Build history of the part. All positions in model axes, mm. A direction names the side the tool comes from. Give positions to 0.01 mm unless a question says otherwise; leave off trailing zeros. Order: outer loops, then holes, each group sorted by start corner. A loop starts at its lowest first (then second) coordinate and runs counter-clockwise, first axis right, second up. Notation, with made-up numbers: (-10, 34.5) - (24, 34.5) arc R17 ccw to (24, 63.5) - close; hole circle Ø1 at (15, 82). An arc over 180 degrees is marked (long way). Use a Markdown table: item, result.
from build123d import *

# Parameters (mm, degrees)
SKETCH_W          = 53.23309
SKETCH_H          = 53.233089
PAD_DEPTH         = 19
SKETCH001_R       = 3.8
POCKET_DEPTH      = 2.001
POCKET_DEPTH_BACK = -17.001
SKETCH002_W       = 57.23309
SKETCH002_H       = 57.233089
SKETCH002_W_2     = 53.23309
SKETCH002_H_2     = 53.233089
PAD001_DEPTH      = 22


with BuildPart() as part:
    # Sketch → Pad (new body)
    with BuildSketch(Plane.XY):
        with Locations((-20.099382, 19.900122)):
            Rectangle(SKETCH_W, SKETCH_H)
    extrude(amount=PAD_DEPTH)

    # Sketch001 (on Sketch) → Pocket (cut, two sides)
    with BuildSketch(Plane.XY.offset(2)) as pocket_sk:
        Circle(SKETCH001_R)
        with Locations((-9.999876, -0.049815)):
            Circle(SKETCH001_R)
        with Locations((-19.999752, -0.09963)):
            Circle(SKETCH001_R)
        with Locations((-29.999628, -0.149445)):
            Circle(SKETCH001_R)
        with Locations((-39.999504, -0.19926)):
            Circle(SKETCH001_R)
        with Locations((-0.049815, 9.999876)):
            Circle(SKETCH001_R)
        with Locations((-10.049691, 9.950061)):
            Circle(SKETCH001_R)
        with Locations((-20.049567, 9.900246)):
            Circle(SKETCH001_R)
        with Locations((-30.049443, 9.850431)):
            Circle(SKETCH001_R)
        with Locations((-40.049319, 9.800616)):
            Circle(SKETCH001_R)
        with Locations((-0.09963, 19.999752)):
            Circle(SKETCH001_R)
        with Locations((-10.099506, 19.949937)):
            Circle(SKETCH001_R)
        with Locations((-20.099382, 19.900122)):
            Circle(SKETCH001_R)
        with Locations((-30.099258, 19.850307)):
            Circle(SKETCH001_R)
        with Locations((-40.099134, 19.800492)):
            Circle(SKETCH001_R)
        with Locations((-0.149445, 29.999628)):
            Circle(SKETCH001_R)
        with Locations((-10.149321, 29.949813)):
            Circle(SKETCH001_R)
        with Locations((-20.149197, 29.899998)):
            Circle(SKETCH001_R)
        with Locations((-30.149073, 29.850183)):
            Circle(SKETCH001_R)
        with Locations((-40.148949, 29.800368)):
            Circle(SKETCH001_R)
        with Locations((-0.19926, 39.999504)):
            Circle(SKETCH001_R)
        with Locations((-10.199136, 39.949689)):
            Circle(SKETCH001_R)
        with Locations((-20.199012, 39.899874)):
            Circle(SKETCH001_R)
        with Locations((-30.198888, 39.850059)):
            Circle(SKETCH001_R)
        with Locations((-40.198764, 39.800244)):
            Circle(SKETCH001_R)
    extrude(amount=-POCKET_DEPTH, mode=Mode.SUBTRACT)
    extrude(pocket_sk.sketch, amount=-POCKET_DEPTH_BACK, mode=Mode.SUBTRACT)

    # Sketch002 → Pad001 (join)
    with BuildSketch(Plane.XY):
        with Locations((-20.099382, 19.900122)):
            Rectangle(SKETCH002_W, SKETCH002_H)
        with Locations((-20.099382, 19.900122)):
            Rectangle(SKETCH002_W_2, SKETCH002_H_2, mode=Mode.SUBTRACT)
    extrude(amount=PAD001_DEPTH)


solid = part.part
1) Slice it at A-A (x = -42.5). Write the cut outline in (y, z).
Computed:
| item | result |
|---|---|
| outline | (-8.72, 0) - (-3.06, 0) - (-3.06, 19) - (-6.72, 19) - (-6.72, 22) - (-8.72, 22) - close; (2.66, 0) - (6.9, 0) - (6.9, 19) - (2.66, 19) - close; (12.7, 0) - (16.86, 0) - (16.86, 19) - (12.7, 19) - close; (22.75, 0) - (26.81, 0) - (26.81, 19) - (22.75, 19) - close; (32.79, 0) - (36.78, 0) - (36.78, 19) - (32.79, 19) - close; (42.82, 0) - (48.52, 0) - (48.52, 22) - (46.52, 22) - (46.52, 19) - (42.82, 19) - close |
2) Two-plate mould, pull along Y, no slides. Class faces 3 (the cylindrical face through (-40.54, 13.57, 9.63)), 4 (the flat face through (-21, 48.517, 11)), 5 (the flat face through (-22, -8, 22)): +Y half, -Y half, draft (parallel to the pull), parting line (faces both ways), or undercut.
Computed:
| item | result |
|---|---|
| face 3 | undercut |
| face 4 | +Y half |
| face 5 | draft |
3) Wall check: line 1 (Y direction, x = -20, z = 5); line 2 (Y direction, x = -40, z = 12); line 3 (X direction, y = 31.5, z = 21). Give the ranges that are in metal, low to high. Write a range as from..to.
Computed:
| item | result |
|---|---|
| line 1 | y = -8.72..-3.9, 3.7..6.1, 13.7..16.1, 23.7..26.1, 33.7..36.11, 43.69..48.52 |
| line 2 | y = -8.72..-4, 3.6..6, 13.6..16, 23.6..26, 33.6..36.01, 43.6..48.52 |
| line 3 | x = -48.72..-46.72, 6.52..8.52 |
4) Pin check, flat tips, straight feed: P1, Ø12, axis at x = -10.2, y = 39.95, coming from the +Z side; P2, Ø6, axis at x = -10.05, y = 9.95, coming from the -Z side. Stop position of each tip, or through.
Computed:
| item | result |
|---|---|
| P1 | stops at z = 19 |
| P2 | passes through |
5) Tool access for faces 1 (the cylindrical face through (-3.796, 0.167, 9.633)), 2 (the flat face through (-46.716, 20, 20)): list every direction of +Z, -Z, +X, -X, +Y, -Y with a clear straight run to the whole face (end or side of a thin tool).
Computed:
| item | result |
|---|---|
| face 1 | +Z, -Z |
| face 2 | +Z |
6) Slice it at C-C (y = -1). Write the cut outline in (x, z).
Computed:
| item | result |
|---|---|
| outline | (-48.72, 0) - (-43.71, 0) - (-43.71, 19) - (-46.72, 19) - (-46.72, 22) - (-48.72, 22) - close; (-36.28, 0) - (-33.7, 0) - (-33.7, 19) - (-36.28, 19) - close; (-26.3, 0) - (-23.69, 0) - (-23.69, 19) - (-26.3, 19) - close; (-16.31, 0) - (-13.68, 0) - (-13.68, 19) - (-16.31, 19) - close; (-6.32, 0) - (-3.67, 0) - (-3.67, 19) - (-6.32, 19) - close; (3.67, 0) - (8.52, 0) - (8.52, 22) - (6.52, 22) - (6.52, 19) - (3.67, 19) - close |
7) Slice it at B-B (z = 15). State how many separate pieces and enclosed holes the cut face has, and give its area (3 significant figures).
Computed:
| item | result |
|---|---|
| separate pieces | 1 |
| enclosed holes | 25 |
| area | 2,140 mm² |
